Geometry: see drawing. Coordinates: mm, zero at the bounding-box minimum. Round coordinates to 2 decimals unless told otherwise and drop trailing zeros. Write each loop counter-clockwise with the first axis right and the second up, starting at its lowest first coordinate (ties: lowest second). Pieces come first, ordered by that corner, then holes. Notation, with made-up numbers: (21.25, 72.5) -> (74.25, 72.5) arc R22 cw to (74.25, 79.5) -> close; hole circle Ø10 at (-27, -26). An arc over 180 degrees is marked (long way). Use CSV: the item, a comma, the result in double quotes.
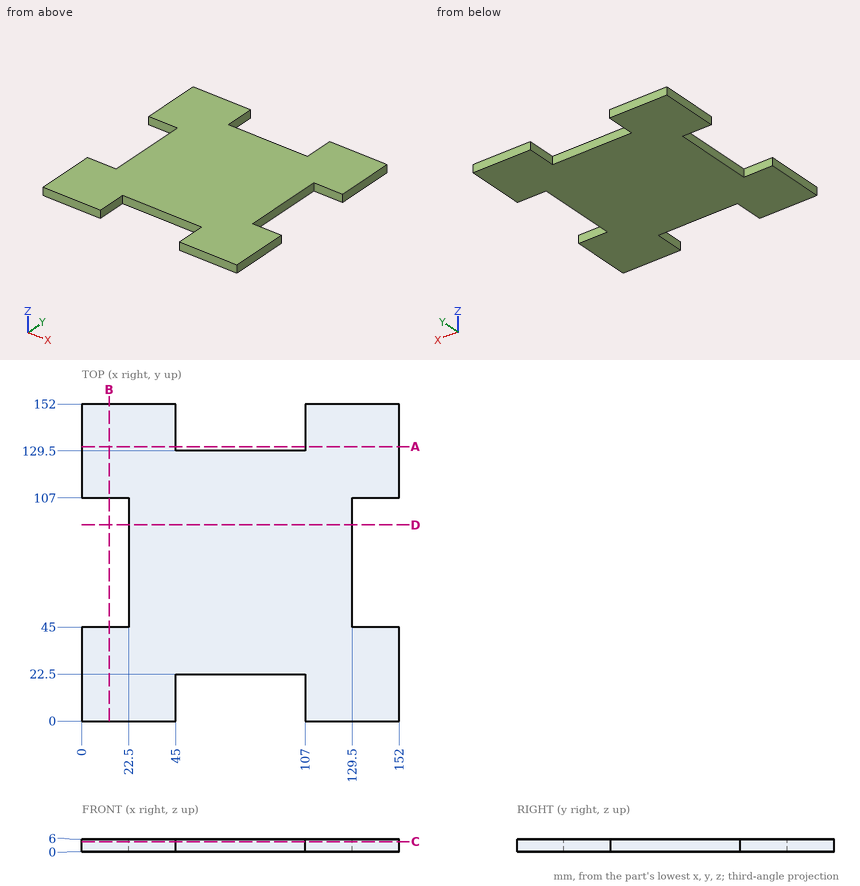
Item 1: Section query A-A on y = 131.5. Return the cut outline in (x, z), plus the area to 3 significant figures.
Worked answers:
outline,"(0, 0) -> (45, 0) -> (45, 6) -> (0, 6) -> close; (107, 0) -> (152, 0) -> (152, 6) -> (107, 6) -> close"
area,"540 mm²"
Item 2: Line query: line 1 (Y direction, x = 9.5, z = 1.3); line 2 (X direction, y = 96, z = 5.05). Output: solid intervals per line, ascending.
Worked answers:
line 1,"y = 0 to 45, 107 to 152"
line 2,"x = 22.5 to 129.5"
Item 3: Section query C-C on z = 4.75. Return the cut outline in (x, y), plus the area to 3 significant figures.
Worked answers:
outline,"(0, 0) -> (45, 0) -> (45, 22.5) -> (107, 22.5) -> (107, 0) -> (152, 0) -> (152, 45) -> (129.5, 45) -> (129.5, 107) -> (152, 107) -> (152, 152) -> (107, 152) -> (107, 129.5) -> (45, 129.5) -> (45, 152) -> (0, 152) -> (0, 107) -> (22.5, 107) -> (22.5, 45) -> (0, 45) -> close"
area,"17,500 mm²"
Item 4: Section query D-D on y = 94. Return the cut outline in (x, z).
Worked answers:
outline,"(22.5, 0) -> (129.5, 0) -> (129.5, 6) -> (22.5, 6) -> close"
Item 5: First-contact query: pin 1 Ø2 at (x, z) = (104.5, 1.5) entering from +Y; pin 2 Ø1.5 at (y, z) = (93, 1) entering from -X; pin 3 Ø1.8 at (x, z) = (91.5, 3.5) entering from -Y. Flat tips, straight axial feed; report the tip coordinate or a pass-through.
Worked answers:
pin 1,"stops at y = 129.5"
pin 2,"stops at x = 22.5"
pin 3,"stops at y = 22.5"
